Geometry check sheet. Reference: the model listing, model coordinates, mm. Face numbers are marked on the shaded views. Round coordinates to 2 decimals unless told otherwise and drop trailing zeros. Order: outer loops, then holes, each group sorted by start corner. A loop starts at its lowest first (then second) coordinate and runs counter-clockwise, first axis right, second up. Notation, with made-up numbers: (52, 35) - (65, 35) arc R23 cw to (65, 60) - close; hole circle Ø1 at (-37, 80.25). An arc over 180 degrees is marked (long way). Return JSON: item names as keys, results as strings. Group by question number.
Q1. Material ranges on line 1 along Y through (x, z) = (-1.65, 0); line 2 along X through (y, z) = (21, -54); line 3 along Y through (x, z) = (-60, -43), recorded low to high.
Q2. Sectioned sample at D-D, the plane z = 23.5. Record the cut outline in (x, y), then the cut area to 3 significant figures.
Q3. Gauge pin test, flat ends, axial feed: pin 1 Ø5 at (x, y) = (-24.5, -9) entering from -Z; pin 2 Ø4 at (y, z) = (0, 16) entering from -X; pin 3 Ø8 at (y, z) = (75.78, -43.75) entering from +X; pin 4 Ø4 at (y, z) = (-75.78, -43.75) entering from -X. Record the tip position at first contact, or that the pin passes through.
Q4. Draft check along Z on the marked faces 1 and 2. Enter one of: pulls with the +Z half, pulls with the -Z half, needs draft (parallel to the pull), parting line crosses it, or undercut.
Q5. Sectioned sample at A-A, the plane x = -57.5. Record the cut outline in (y, z), then the cut area to 3 significant figures.
Q6. Sectioned sample at B-B, the plane z = -9.5. Record the cut outline in (x, y).
Q7. Sectioned sample at C-C, the plane y = 37. Record the cut outline in (x, z).
```python
from build123d import *

# Parameters (mm, degrees)
SKETCH3_R           = 12.5
CUT_EXTRUDE2_DEPTH  = 30
SKETCH4_R           = 5
BOSS_EXTRUDE1_DEPTH = 15
SKETCH5_R           = 2.5
CUT_EXTRUDE3_DEPTH  = 10.5
CIRPATTERN1_COUNT   = 3
CHAMFER1_SIZE       = 10
CHAMFER2_SIZE       = 10
CHAMFER3_SIZE       = 10
SKETCH6_R           = 1.75
CUT_EXTRUDE4_DEPTH  = 10.5
SKETCH7_R           = 2.5
CUT_EXTRUDE5_DEPTH  = 10.5
CIRPATTERN2_COUNT   = 3


with BuildPart() as part:
    # Sketch1 → Revolve1 (revolve)
    with BuildSketch(Plane(origin=(0, 0, 0), x_dir=(-1, 0, 0), z_dir=(0, 1, 0)), mode=Mode.PRIVATE) as revolve1_sk:
        Polygon((0, 0), (0, 87.5), (65.6, 87.5), (65.6, 81.5), (6, 81.5), (6, 0), align=None)
    revolve(revolve1_sk.sketch.rotate(Axis((38.11091851, 0, 0), (-1, 0, 0)), 180), axis=Axis((38.11091851, 0, 0), (-1, 0, 0)))

    # Sketch3 → Cut-Extrude2 (cut)
    with BuildSketch(Plane.YZ):
        with Locations(Location((0, 0, 0), (0, 0, 270))):
            Circle(SKETCH3_R)
    extrude(amount=-CUT_EXTRUDE2_DEPTH, mode=Mode.SUBTRACT)

    # Sketch4 → Boss-Extrude1 (add)
    with BuildSketch(Plane(origin=(-65.6, 0, 0), x_dir=(0, -1, 0), z_dir=(-1, 0, 0))):
        with Locations((0, 87.5)):
            Circle(SKETCH4_R)
        with Locations((-75.777222831, -43.75)):
            Circle(SKETCH4_R)
        with Locations((75.777222831, -43.75)):
            Circle(SKETCH4_R)
    extrude(amount=-BOSS_EXTRUDE1_DEPTH)

    # Sketch5 → Cut-Extrude3 (cut)
    with BuildSketch(Plane(origin=(-65.6, 0, 0), x_dir=(0, -1, 0), z_dir=(-1, 0, 0))):
        with Locations(Location((0, 87.5, 0), (0, 0, 90))):
            Circle(SKETCH5_R)
    cut_extrude3 = extrude(amount=-CUT_EXTRUDE3_DEPTH, mode=Mode.SUBTRACT)

    # CirPattern1: Cut-Extrude3 ×3 about axis
    cirpattern1_axis = Axis((0, 0, 0), (1, 0, 0))
    for i in range(1, CIRPATTERN1_COUNT):
        add(cut_extrude3.rotate(cirpattern1_axis, i * 360 / CIRPATTERN1_COUNT), mode=Mode.SUBTRACT)

    # Chamfer1
    # the kernel refuses this chamfer: 10 mm, written as the material it adds along each edge
    with BuildSketch(Plane(origin=(-50.6, 0, 0), x_dir=(0, 0.9851517122975438, -0.17168606162766187), z_dir=(0, 0.17168606162766187, 0.9851517122975438))) as chamfer1_piece_1_section:
        Polygon((87.5, -CHAMFER1_SIZE), (87.5 + CHAMFER1_SIZE, 0), (87.5, 0), align=None)
    chamfer1_piece_1 = revolve(axis=Axis((-50.6, 0, 0), (-1, 0, 0)), revolution_arc=40.228270546, mode=Mode.PRIVATE)
    chamfer1_piece_1 = chamfer1_piece_1 & Plane(origin=(-46.494939835, 75.777222831, -43.75), x_dir=(0, -1, 0), z_dir=(-1, 0, 0)) * Cylinder(5, 390, mode=Mode.PRIVATE)
    add(chamfer1_piece_1)

    # Chamfer2
    # the kernel refuses this chamfer: 10 mm, written as the material it adds along each edge
    with BuildSketch(Plane(origin=(-50.6, 0, 0), x_dir=(0, -0.3438913653035208, 0.9390094402452408), z_dir=(0, -0.9390094402452408, -0.3438913653035208))) as chamfer2_piece_1_section:
        Polygon((87.5, -CHAMFER2_SIZE), (87.5 + CHAMFER2_SIZE, 0), (87.5, 0), align=None)
    chamfer2_piece_1 = revolve(axis=Axis((-50.6, 0, 0), (-1, 0, 0)), revolution_arc=40.228270546, mode=Mode.PRIVATE)
    chamfer2_piece_1 = chamfer2_piece_1 & Plane(origin=(-46.494939444, 0, 87.5), x_dir=(0, -1, 0), z_dir=(-1, 0, 0)) * Cylinder(5, 390, mode=Mode.PRIVATE)
    add(chamfer2_piece_1)

    # Chamfer3
    # the kernel refuses this chamfer: 10 mm, written as the material it adds along each edge
    with BuildSketch(Plane(origin=(-50.6, 0, 0), x_dir=(0, -0.6412603469940208, -0.7673233786175866), z_dir=(0, 0.7673233786175866, -0.6412603469940208))) as chamfer3_piece_1_section:
        Polygon((87.5, -CHAMFER3_SIZE), (87.5 + CHAMFER3_SIZE, 0), (87.5, 0), align=None)
    chamfer3_piece_1 = revolve(axis=Axis((-50.6, 0, 0), (-1, 0, 0)), revolution_arc=40.228270546, mode=Mode.PRIVATE)
    chamfer3_piece_1 = chamfer3_piece_1 & Plane(origin=(-46.494939164, -75.777222831, -43.75), x_dir=(0, -1, 0), z_dir=(-1, 0, 0)) * Cylinder(5, 390, mode=Mode.PRIVATE)
    add(chamfer3_piece_1)

    # Sketch6 → Cut-Extrude4 (cut)
    with BuildSketch(Plane.YZ):
        with Locations(Location((-16, 0, 0), (0, 0, 270))):
            Circle(SKETCH6_R)
        with Locations(Location((16, 0, 0), (0, 0, 270))):
            Circle(SKETCH6_R)
        with Locations(Location((0, 16, 0), (0, 0, 270))):
            Circle(SKETCH6_R)
        with Locations(Location((0, -16, 0), (0, 0, 270))):
            Circle(SKETCH6_R)
    extrude(amount=-CUT_EXTRUDE4_DEPTH, mode=Mode.SUBTRACT)

    # Sketch7 → Cut-Extrude5 (cut)
    with BuildSketch(Plane.YZ):
        with Locations(Location((0, 35, 0), (0, 0, 270))):
            Circle(SKETCH7_R)
    cut_extrude5 = extrude(amount=-CUT_EXTRUDE5_DEPTH, mode=Mode.SUBTRACT)

    # CirPattern2: Cut-Extrude5 ×3 about axis
    cirpattern2_axis = Axis((0, 0, 0), (1, 0, 0))
    for i in range(1, CIRPATTERN2_COUNT):
        add(cut_extrude5.rotate(cirpattern2_axis, i * 360 / CIRPATTERN2_COUNT), mode=Mode.SUBTRACT)


solid = part.part
```
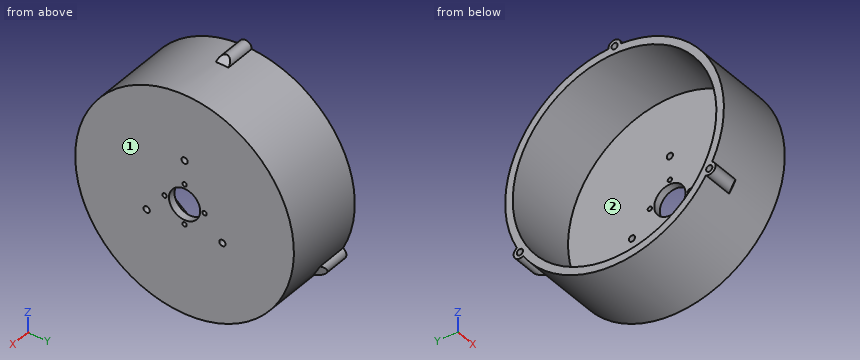
Reply:
{
 "1": {"line 1": "-87.5 to -17.75, -14.25 to -12.5, 12.5 to 14.25, 17.75 to 87.5", "line 2": "-6 to 0", "line 3": "-80.72 to -78.16, -73.39 to -69.23, 69.23 to 73.39, 78.16 to 80.72"},
 "2": {"outline": "(-65.6, -84.29) - (0, -84.29) - (0, 84.29) - (-65.6, 84.29) - (-65.6, 78.04) - (-6, 78.04) - (-6, -78.04) - (-65.6, -78.04) - close", "area": "1,760 mm^2"},
 "3": {"pin 1": "z = -87.26", "pin 2": "x = -6", "pin 3": "x = 0", "pin 4": "x = -55.1"},
 "4": {"face 1": "needs draft", "face 2": "undercut"},
 "5": {"outline": "(-78.15, -39.35) arc R5 ccw (long way) to (-73.15, -48.01) arc R87.5 ccw to (73.15, -48.01) arc R5 ccw (long way) to (78.15, -39.35) arc R87.5 ccw to (5, 87.36) arc R5 ccw (long way) to (-5, 87.36) arc R87.5 ccw to start; hole circle Ø163 at (0, 0); hole circle Ø5 at (-75.78, -43.75); hole circle Ø5 at (0, 87.5); hole circle Ø5 at (75.78, -43.75)", "area": "3,250 mm^2"},
 "6": {"outline": "(-65.6, -86.98) - (0, -86.98) - (0, -8.12) - (-6, -8.12) - (-6, -80.94) - (-65.6, -80.94) - close; (-65.6, 80.94) - (-6, 80.94) - (-6, 8.12) - (0, 8.12) - (0, 86.98) - (-65.6, 86.98) - close"},
 "7": {"outline": "(-65.6, -79.29) - (0, -79.29) - (0, 79.29) - (-65.6, 79.29) - (-65.6, 72.62) - (-6, 72.62) - (-6, -72.62) - (-65.6, -72.62) - close"}
}
